Can you work these out from the model? Positions are in its coordinate system, mm. A direction names the side the tool comes from. Coordinates: 2 decimals unless noted, no trailing zeros. Loops run counter-clockwise (first coordinate to the right, second up) from the corner with the lowest first, then second, coordinate; pieces in that order, holes last.
```python
from build123d import *

# Parameters (mm, degrees)
F2_R        = 10
F3_DEPTH    = 1.5875
F4_T1_DEPTH = 3.175


# Not quite as in the source:
# - a fillet or chamfer that OpenCascade refuses, or shapes differently, is made with other operations: its cross-section is extruded or revolved along the edge and cut away or added


with BuildPart() as f3:
    # F2 (on Top) → F3 (new body, symmetric)
    with BuildSketch(Plane.XY):
        with BuildLine():
            ThreePointArc((7.7459666924, 14), (13.7828782748, 19.8739759746), (16, 28))
            ThreePointArc((16, 28), (-8.1260240254, 41.7828782748), (-7.7459666924, 14))
            ThreePointArc((-7.7459666924, 14), (0, 16), (7.7459666924, 14))
        make_face()
        with Locations((0, 28)):
            Circle(F2_R, mode=Mode.SUBTRACT)
        with BuildLine():
            ThreePointArc((7.7459666924, 14), (0, 12), (-7.7459666924, 14))
            ThreePointArc((-7.7459666924, 14), (-13.8564064606, 8), (-15.9973389992, -0.2917960675))
            ThreePointArc((-15.9973389992, -0.2917960675), (-10.3923048454, -6), (-8.2513723068, -13.7082039325))
            ThreePointArc((-8.2513723068, -13.7082039325), (0, -16), (8.2513723068, -13.7082039325))
            ThreePointArc((8.2513723068, -13.7082039325), (10.3923048454, -6), (15.9973389992, -0.2917960675))
            ThreePointArc((15.9973389992, -0.2917960675), (15.999334736, -0.1459041003), (16, 0))
            ThreePointArc((16, 0), (13.7828782748, 8.1260240254), (7.7459666924, 14))
        make_face()
        Circle(F2_R, mode=Mode.SUBTRACT)
        with BuildLine():
            ThreePointArc((-8.2513723068, -13.7082039325), (-13.8564064606, -8), (-15.9973389992, -0.2917960675))
            ThreePointArc((-15.9973389992, -0.2917960675), (-38.1774936811, -21.8733107106), (-8.248711306, -14))
            ThreePointArc((-8.248711306, -14), (-8.24937657, -13.8540958997), (-8.2513723068, -13.7082039325))
        make_face()
        with Locations((-24.248711306, -14)):
            Circle(F2_R, mode=Mode.SUBTRACT)
        with BuildLine():
            ThreePointArc((-8.2513723068, -13.7082039325), (-10.3923048454, -6), (-15.9973389992, -0.2917960675))
            ThreePointArc((-15.9973389992, -0.2917960675), (-13.8564064606, -8), (-8.2513723068, -13.7082039325))
        make_face()
        with BuildLine():
            ThreePointArc((7.7459666924, 14), (0, 16), (-7.7459666924, 14))
            ThreePointArc((-7.7459666924, 14), (0, 12), (7.7459666924, 14))
        make_face()
        with BuildLine():
            ThreePointArc((8.2513723068, -13.7082039325), (13.8564064606, -8), (15.9973389992, -0.2917960675))
            ThreePointArc((15.9973389992, -0.2917960675), (10.3923048454, -6), (8.2513723068, -13.7082039325))
        make_face()
        with BuildLine():
            ThreePointArc((40.248711306, -14), (32.1220220166, -0.0712176249), (15.9973389992, -0.2917960675))
            ThreePointArc((15.9973389992, -0.2917960675), (13.8564064606, -8), (8.2513723068, -13.7082039325))
            ThreePointArc((8.2513723068, -13.7082039325), (24.1028072057, -29.999334736), (40.248711306, -14))
        make_face()
        with Locations((24.248711306, -14)):
            Circle(F2_R, mode=Mode.SUBTRACT)
    extrude(amount=F3_DEPTH, both=True)

    # F4: fillet of radius 13 on 6 edges, made by hand

    # F4_s2 → F4_t1 (join)
    with BuildSketch(Plane.XY.offset(-1.5875)):
        with BuildLine():
            ThreePointArc((14.0120552819, 20.275862069), (12.3968501984, 14), (14.0120552819, 7.724137931))
            ThreePointArc((14.0120552819, 7.724137931), (11.3225214169, 11.3048887108), (7.7459666924, 14))
            ThreePointArc((7.7459666924, 14), (11.3225214169, 16.6951112892), (14.0120552819, 20.275862069))
        make_face()
        with BuildLine():
            ThreePointArc((13.6953273115, 8.2727268678), (18.3227807522, 3.7359871987), (24.5654392763, 1.9968647989))
            ThreePointArc((24.5654392763, 1.9968647989), (20.1196512039, 1.4580355373), (15.9973389992, -0.2917960675))
            ThreePointArc((15.9973389992, -0.2917960675), (15.451581519, 4.1531468265), (13.6953273115, 8.2727268678))
        make_face()
        with BuildLine():
            ThreePointArc((10.5533839944, -22.2727268678), (5.9259305538, -17.7359871987), (-0.3167279703, -15.9968647989))
            ThreePointArc((-0.3167279703, -15.9968647989), (4.1290601021, -15.4580355373), (8.2513723068, -13.7082039325))
            ThreePointArc((8.2513723068, -13.7082039325), (8.797129787, -18.1531468265), (10.5533839944, -22.2727268678))
        make_face()
        with BuildLine():
            ThreePointArc((0.3167279703, -15.9968647989), (-5.9259305538, -17.7359871987), (-10.5533839944, -22.2727268678))
            ThreePointArc((-10.5533839944, -22.2727268678), (-8.797129787, -18.1531468265), (-8.2513723068, -13.7082039325))
            ThreePointArc((-8.2513723068, -13.7082039325), (-4.1290601021, -15.4580355373), (0.3167279703, -15.9968647989))
        make_face()
        with BuildLine():
            ThreePointArc((-24.5654392763, 1.9968647989), (-18.3227807522, 3.7359871987), (-13.6953273115, 8.2727268678))
            ThreePointArc((-13.6953273115, 8.2727268678), (-15.451581519, 4.1531468265), (-15.9973389992, -0.2917960675))
            ThreePointArc((-15.9973389992, -0.2917960675), (-20.1196512039, 1.4580355373), (-24.5654392763, 1.9968647989))
        make_face()
        with BuildLine():
            ThreePointArc((-14.0120552819, 20.275862069), (-12.3968501984, 14), (-14.0120552819, 7.724137931))
            ThreePointArc((-14.0120552819, 7.724137931), (-11.3225214169, 11.3048887108), (-7.7459666924, 14))
            ThreePointArc((-7.7459666924, 14), (-11.3225214169, 16.6951112892), (-14.0120552819, 20.275862069))
        make_face()
    extrude(amount=F4_T1_DEPTH)


solid = f3.part
```
Item 1: On a 3-axis mill with a long thin cutter (end or side, diameter ignored), from which of +Z, -Z, +X, -X, +Y, -Y can I reach the whole of each face in a straight line? I mean faces 1 (the face through (18.383, 3.702, -0.022)), 2 (the face through (6.14, -17.86, -0.02)), 3 (the face through (-2.17, -9.76, -0.02)), 4 (the face through (9.132, 4.432, 1.588)), 5 (the face through (-18.539, 3.614, -0.022)). Say none if no direction works.
Results are:
face 1: +Z, -Z, +X
face 2: +Z, -Z, -Y
face 3: +Z, -Z
face 4: +Z, +X, -X, +Y, -Y
face 5: +Z, -Z, -X
Item 2: Suppose I cut it at A-A, the plane y = 28. Please give me the cut outline in (x, z).
Results are:
outline: (-16, -1.59) - (-10, -1.59) - (-10, 1.59) - (-16, 1.59) - close; (10, -1.59) - (16, -1.59) - (16, 1.59) - (10, 1.59) - close
Item 3: Suppose I cut it at B-B, the plane z = -0.95. Please give me the cut outline in (x, y).
Results are:
outline: (-24.57, 2) arc R16 ccw (long way) to (-10.55, -22.27) arc R13 cw to (0, -16.01) arc R13 cw to (10.55, -22.27) arc R16 ccw (long way) to (24.57, 2) arc R13 cw to (13.86, 8) arc R13 cw to (14.01, 20.28) arc R16 ccw (long way) to (-14.01, 20.28) arc R13 cw to (-13.86, 8) arc R13 cw to start; hole circle Ø20 at (-24.25, -14); hole circle Ø20 at (0, 0); hole circle Ø20 at (0, 28); hole circle Ø20 at (24.25, -14)
Item 4: I'm going to push flat-ended pins straight in: P1, Ø12, axis at x = -24.25, y = -14, coming from the +Z side (3 decimals); P2, Ø1, axis at x = -3.5, z = -1, coming from the +Y side; P3, Ø1.5, axis at y = -22.5, z = 0.5, coming from the +X side. Where does each tip first touch, or does it pass through?
Results are:
P1: passes through
P2: stops at y = 43.72
P3: stops at x = 38.25
Item 5: We'd pull the mould along X, two halves only. Please class faces 6 (the face through (37.867, -22.399, 0.022)), 7 (the face through (-12.4, 14.2, 0)), 8 (the face through (12.4, 14.2, 0)): +X half, -X half, draft (parallel to the pull), parting line (faces both ways), or undercut.
Results are:
face 6: undercut
face 7: -X half
face 8: +X half
Item 6: Suppose I cut it at C-C, the plane x = 27. Please give me the cut outline in (y, z).
Results are:
outline: (-29.76, -1.59) - (-23.61, -1.59) - (-23.61, 1.59) - (-29.76, 1.59) - close; (-4.39, -1.59) - (1.76, -1.59) - (1.76, 1.59) - (-4.39, 1.59) - close
Item 7: Suppose I cut it at D-D, the plane x = -7. Please give me the cut outline in (y, z).
Results are:
outline: (-18.43, -1.59) - (-7.14, -1.59) - (-7.14, 1.59) - (-18.43, 1.59) - close; (7.14, -1.59) - (20.86, -1.59) - (20.86, 1.59) - (7.14, 1.59) - close; (35.14, -1.59) - (42.39, -1.59) - (42.39, 1.59) - (35.14, 1.59) - close
Item 8: I need wall thicknesses on line 1 along Y through (x, z) = (3.5, -1.1); line 2 along X through (y, z) = (-9, 0.6); line 3 along Y through (x, z) = (21, -0.2). Which ranges of each line are inside material? Lowest first, please.
Results are:
line 1: y = -16.65 to -9.37, 9.37 to 18.63, 37.37 to 43.61
line 2: x = -39.45 to -32.91, -15.59 to -4.36, 4.36 to 15.59, 32.91 to 39.45
line 3: y = -29.67 to -23.46, -4.54 to 2.57
